Check sheet for the modelled part. Datum: model origin and axes. Units: mm. Coordinates: 2 decimals unless noted, no trailing zeros. Order: outer loops, then holes, each group sorted by start corner. A loop starts at its lowest first (then second) coordinate and runs counter-clockwise, first axis right, second up.
Autodesk Fusion 360 part; units mm, degrees
sketch "Sketch1" plane through (0, 0, 0) normal (1, 0, 0) x (0, 1, 0)
  circle A0 centre (0, 0) radius 5
  line L0 (0, 5) -> (80, 5)
  line L1 (0, -5) -> (80, -5)
  circle A1 centre (80, 0) radius 5
  dimension "d1" = 10
  dimension "d2" = 80
extrude "Extrude1" add sketch "Sketch1" along normal blind 4
sketch "Sketch2" plane through (4, 0, 0) normal (1, 0, 0) x (0, 1, 0)
  arc A0 (0, 5) -> (0, -5) centre (0, 0) ccw
  line L0 (0, -5) -> (80, -5)
  arc A1 (80, -5) -> (80, 5) centre (80, 0) ccw
  line L1 (80, 5) -> (0, 5)
  circle A2 centre (0, 0) radius 2
  circle A3 centre (80, 0) radius 2
  dimension "d5" = 4
  dimension "d6" = 4
extrude "Extrude2" cut sketch "Sketch2" against normal blind 20 contours A2 | A3
sketch "Sketch3" plane through (4, 0, 0) normal (1, 0, 0) x (0, 1, 0)
  circle A0 centre (0, 0) radius 2
  circle A1 centre (80, 0) radius 2
  arc A2 (0, 5) -> (0, -5) centre (0, 0) ccw
  line L0 (0, -5) -> (80, -5)
  arc A3 (80, -5) -> (80, 5) centre (80, 0) ccw
  line L1 (80, 5) -> (0, 5)
  circle A4 centre (40, 0) radius 2
  dimension "d9" = 4
extrude "Extrude3" cut sketch "Sketch3" against normal blind 20 contours A4
sketch "Sketch4" plane through (0, 0, 0) normal (0, 0, 1) x (1, 0, 0)
sketch "Sketch5" plane through (4, 0, 0) normal (1, 0, 0) x (0, 1, 0)
  circle A0 centre (40, 0) radius 2
  circle A1 centre (0, 0) radius 2
  circle A2 centre (80, 0) radius 2
  arc A3 (0, 5) -> (0, -5) centre (0, 0) ccw
  line L0 (0, -5) -> (80, -5)
  arc A4 (80, -5) -> (80, 5) centre (80, 0) ccw
  line L1 (80, 5) -> (0, 5)
(1) Thickness scan on probe 1 along Z at (x, y) = (0.95, 80); probe 2 along Z at (x, y) = (1.5, 1.5); probe 3 along Y at (x, z) = (1.1, 0.75). Record the ranges inside material, lowest first.
Filled in:
probe 1: z = -5 to -2, 2 to 5
probe 2: z = -5 to -1.32, 1.32 to 5
probe 3: y = -4.94 to -1.85, 1.85 to 38.15, 41.85 to 78.15, 81.85 to 84.94
(2) Cross-section at C-C (y = 40). Enter the section's corners in (x, z), and give its area (3 significant figures).
Filled in:
outline: (0, -5) - (4, -5) - (4, -2) - (0, -2) - close; (0, 2) - (4, 2) - (4, 5) - (0, 5) - close
area: 24.0 mm2
(3) Cross-section at D-D (z = -4.25). Enter the section's corners in (x, y).
Filled in:
outline: (0, -2.63) - (4, -2.63) - (4, 82.63) - (0, 82.63) - close
(4) Release check for a two-part mould opening along Y. For faces 1 (the cylindrical face through (2, 0, -2)), 2 (the cylindrical face through (2, -5, 0)), 3 (the flat face through (2, 39, -5)) record: +Y half, -Y half, draft (parallel to the pull), parting line (faces both ways), or undercut.
Filled in:
face 1: undercut
face 2: -Y half
face 3: draft
(5) Cross-section at A-A (z = 0). Enter the section's corners in (x, y).
Filled in:
outline: (0, -5) - (4, -5) - (4, -2) - (0, -2) - close; (0, 2) - (4, 2) - (4, 38) - (0, 38) - close; (0, 42) - (4, 42) - (4, 78) - (0, 78) - close; (0, 82) - (4, 82) - (4, 85) - (0, 85) - close
(6) Cross-section at B-B (x = 1.1). Enter the section's corners in (y, z), and give its area (3 significant figures).
Filled in:
outline: (0, -5) - (80, -5) arc R5 ccw to (80, 5) - (0, 5) arc R5 ccw to start; hole circle Ø4 at (0, 0); hole circle Ø4 at (40, 0); hole circle Ø4 at (80, 0)
area: 841 mm2
